Design review of the part built by this model. Coordinates are the model's own, in mm. Face numbers are marked on the shaded views. A direction names the side the tool comes from. Coordinates: 2 decimals unless noted, no trailing zeros. Write each loop counter-clockwise with the first axis right and the second up, starting at its lowest first coordinate (ties: lowest second). Pieces come first, ordered by that corner, then holes. Notation, with made-up numbers: (-17.75, 12.5) - (2.25, 12.5) arc R27 ccw to (2.25, 50.5) - close; hole circle Ø7 at (89, 8). An arc over 180 degrees is marked (long way). Answer as a JSON object with one key per item and string values.
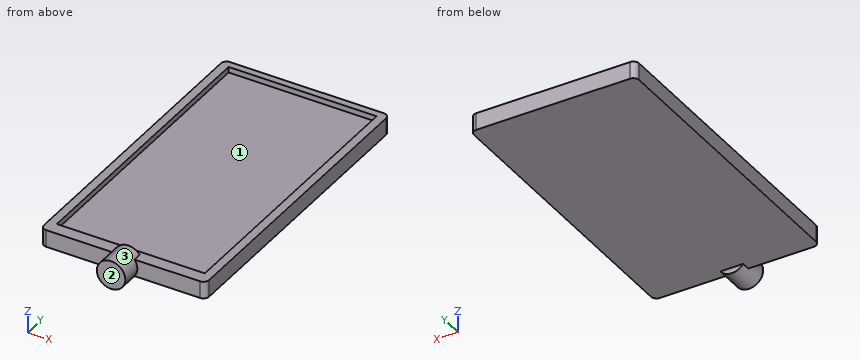
```python
from build123d import *

# Parameters (mm, degrees)
SKETCH007_R       = 2.5
PAD006_DEPTH      = 5
SKETCH008_W       = 29
SKETCH008_H       = 3
PAD007_DEPTH      = 52
PAD007_DEPTH_BACK = 1.5
FILLET_R          = 1
SKETCH010_W       = 26
SKETCH010_H       = 50
POCKET001_DEPTH   = 1


with BuildPart() as part:
    # Sketch007 (on Face1 of CopyPad001) → Pad006 (new body)
    with BuildSketch(Plane(origin=(0, 17.25, 0), x_dir=(-1, 0, 0), z_dir=(0, 1, 0))):
        with Locations((0, -4)):
            Circle(SKETCH007_R)
    extrude(amount=PAD006_DEPTH)

    # Sketch008 (on Face3 of Pad006) → Pad007 (join, two sides)
    with BuildSketch(Plane(origin=(0, 22.25, 0), x_dir=(-1, 0, 0), z_dir=(0, 1, 0))) as pad007_sk:
        with Locations((0, -4)):
            Rectangle(SKETCH008_W, SKETCH008_H)
    extrude(amount=PAD007_DEPTH)
    extrude(pad007_sk.sketch, amount=-PAD007_DEPTH_BACK)

    # Fillet
    fillet_edges = [part.edges().sort_by_distance(p)[0] for p in [
        (14.5, 74.25, -4),
        (14.5, 20.75, -4),
        (-14.5, 74.25, -4),
        (-14.5, 20.75, -4),
    ]]
    fillet(fillet_edges, radius=FILLET_R)

    # Sketch010 (on Face5 of Fillet) → Pocket001 (cut)
    with BuildSketch(Plane.XY.offset(-2.5)):
        with Locations((0, 48)):
            Rectangle(SKETCH010_W, SKETCH010_H)
    extrude(amount=-POCKET001_DEPTH, mode=Mode.SUBTRACT)


solid = part.part
```
(1) Take a section at D-D, the plane x = -6.5. Write out the cut boundary in (y, z).
Solved:
{"outline": "(20.75, -5.5) - (74.25, -5.5) - (74.25, -2.5) - (73, -2.5) - (73, -3.5) - (23, -3.5) - (23, -2.5) - (20.75, -2.5) - close"}
(2) For pin 1 (6 mm diameter, centred on x = -7, y = 58.5, fed in from -Z); pin 2 (2 mm diameter, centred on x = 7.5, y = 55, fed in from +Z); pin 3 (0.5 mm diameter, centred on x = 4, z = -3, fed in from -Y), all flat-tipped, find the tip position at first contact; note any pin that passes through.
Solved:
{"pin 1": "stops at z = -5.5", "pin 2": "stops at z = -3.5", "pin 3": "stops at y = 20.75"}
(3) Tool access review of the marked faces 1, 2 and 3: name each direction out of +Z, -Z, +X, -X, +Y, -Y from which nothing blocks a thin tool from reaching the whole face with its end or side.
Solved:
{"face 1": "+Z", "face 2": "+Z, -Z, +X, -X, -Y", "face 3": "-Y"}
(4) Take a section at A-A, the plane x = 0. Write out the cut boundary in (y, z), and give its area (3 significant figures).
Solved:
{"outline": "(17.25, -6.5) - (22.25, -6.5) - (22.25, -5.5) - (74.25, -5.5) - (74.25, -2.5) - (73, -2.5) - (73, -3.5) - (23, -3.5) - (23, -2.5) - (22.25, -2.5) - (22.25, -1.5) - (17.25, -1.5) - close", "area": "131 mm^2"}
(5) To check wall thickness, follow line 1 (Y direction, x = 6.75, z = -3.45); line 2 (X direction, y = 49.5, z = -3.05); line 3 (Y direction, x = -1.75, z = -2.8). State the ranges of each line that lie inside material, in increasing order. Write a range as from..to.
Solved:
{"line 1": "y = 20.75..23, 73..74.25", "line 2": "x = -14.5..-13, 13..14.5", "line 3": "y = 17.25..23, 73..74.25"}
(6) Take a section at C-C, the plane z = -4.9. Write out the cut boundary in (x, y).
Solved:
{"outline": "(-14.5, 21.75) arc R1 ccw to (-13.5, 20.75) - (-2.33, 20.75) - (-2.33, 17.25) - (2.33, 17.25) - (2.33, 20.75) - (13.5, 20.75) arc R1 ccw to (14.5, 21.75) - (14.5, 73.25) arc R1 ccw to (13.5, 74.25) - (-13.5, 74.25) arc R1 ccw to (-14.5, 73.25) - close"}
(7) Take a section at B-B, the plane y = 29.5. Write out the cut boundary in (x, z).
Solved:
{"outline": "(-14.5, -5.5) - (14.5, -5.5) - (14.5, -2.5) - (13, -2.5) - (13, -3.5) - (-13, -3.5) - (-13, -2.5) - (-14.5, -2.5) - close"}
